Check sheet for the modelled part. Datum: model origin and axes. Units: mm. Face numbers are marked on the shaded views. A direction names the side the tool comes from. Give positions to 0.01 mm unless a question says otherwise; leave off trailing zeros. Write each loop counter-clockwise with the first axis right and the second up, starting at its lowest first coordinate (ties: lowest second). Pieces come first, ordered by that corner, then holes. Notation, with made-up numbers: (73, -0.5) -> (126, -0.5) arc R26 ccw to (126, 20.5) -> close; hole circle Ø7 at (-25, 89.25). An arc over 180 degrees is marked (long way). Answer as a JSON object with one key per item and string values.
from build123d import *

# Parameters (mm, degrees)
BOSS_EXTRUDE1_DEPTH = 19.05
SKETCH2_R           = 2
CUT_EXTRUDE1_DEPTH  = 10.16
SKETCH3_W           = 7.62
SKETCH3_H           = 3.81
CUT_EXTRUDE2_DEPTH  = 64.697811893


with BuildPart() as part:
    # Sketch1 → Boss-Extrude1 (new, symmetric)
    with BuildSketch(Plane.XY):
        with BuildLine():
            Line((-22.352, 0), (-22.352, 17.272))
            Line((-22.352, 17.272), (-19.812, 17.272))
            Line((-19.812, 17.272), (-19.812, 21.082))
            Line((-19.812, 21.082), (-28.702, 21.082))
            Line((-28.702, 21.082), (-28.702, 17.272))
            Line((-28.702, 17.272), (-26.162, 17.272))
            Line((-26.162, 17.272), (-26.162, 0))
            ThreePointArc((-26.162, 0), (0, -26.162), (26.162, 0))
            Line((26.162, 0), (26.162, 17.272))
            Line((26.162, 17.272), (28.702, 17.272))
            Line((28.702, 17.272), (28.702, 21.082))
            Line((28.702, 21.082), (19.812, 21.082))
            Line((19.812, 21.082), (19.812, 17.272))
            Line((19.812, 17.272), (22.352, 17.272))
            Line((22.352, 17.272), (22.352, 0))
            ThreePointArc((22.352, 0), (0, -22.352), (-22.352, 0))
        make_face()
    extrude(amount=BOSS_EXTRUDE1_DEPTH, both=True)

    # Sketch2 → Cut-Extrude1 (cut)
    with BuildSketch(Plane(origin=(0, 21.082, 0), x_dir=(1, 0, 0), z_dir=(0, 1, 0))):
        with Locations(Location((-24.257, 12.7, 0), (0, 0, 270))):
            Circle(SKETCH2_R)
        with Locations(Location((-24.257, -12.7, 0), (0, 0, 270))):
            Circle(SKETCH2_R)
        with Locations(Location((24.257, -12.7, 0), (0, 0, 270))):
            Circle(SKETCH2_R)
        with Locations(Location((24.257, 12.7, 0), (0, 0, 270))):
            Circle(SKETCH2_R)
    extrude(amount=-CUT_EXTRUDE1_DEPTH, mode=Mode.SUBTRACT)

    # Sketch3 → Cut-Extrude2 (cut, through all)
    with BuildSketch(Plane.ZY.offset(26.162)):
        with Locations((-12.7, 15.367)):
            Rectangle(SKETCH3_W, SKETCH3_H)
        with Locations((12.7, 15.367)):
            Rectangle(SKETCH3_W, SKETCH3_H)
    extrude(amount=-CUT_EXTRUDE2_DEPTH, mode=Mode.SUBTRACT)


solid = part.part
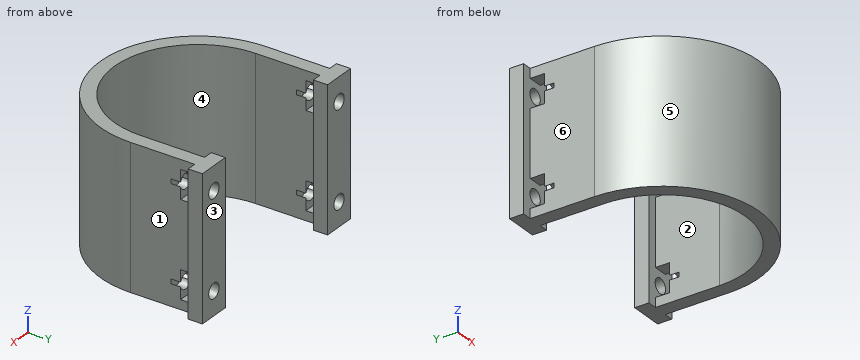
1. Sectioned sample at C-C, the plane x = -20.5. Enter the section's corners in (y, z).
Determined:
{"outline": "(-16.25, -19.05) -> (-8.91, -19.05) -> (-8.91, 19.05) -> (-16.25, 19.05) -> close; (17.27, -19.05) -> (21.08, -19.05) -> (21.08, 19.05) -> (17.27, 19.05) -> close"}
2. Access from +Z, -Z, +X, -X, +Y, -Y to the whole of each face (thin tool, end or side, straight path). Record for the marked faces 1, 2 and 3.
Determined:
{"face 1": "+Z, -Z, +X, -Y", "face 2": "+Z, -Z", "face 3": "+Z, -Z, +X, -X, +Y"}
3. Sectioned sample at A-A, the plane y = 6.5. Enter the section's corners in (x, z), plus the area to 3 significant figures.
Determined:
{"outline": "(-26.16, -19.05) -> (-22.35, -19.05) -> (-22.35, 19.05) -> (-26.16, 19.05) -> close; (22.35, -19.05) -> (26.16, -19.05) -> (26.16, 19.05) -> (22.35, 19.05) -> close", "area": "290 mm^2"}
4. Sectioned sample at D-D, the plane x = 0. Enter the section's corners in (y, z), plus the area to 3 significant figures.
Determined:
{"outline": "(-26.16, -19.05) -> (-22.35, -19.05) -> (-22.35, 19.05) -> (-26.16, 19.05) -> close", "area": "145 mm^2"}
5. Mould release check, pull along X, two halves, no side actions. Record for the marked faces 4, 5 and 6: released by +X, released by -X, zero draft, split by the parting line, or undercut.
Determined:
{"face 4": "undercut", "face 5": "split by the parting line", "face 6": "released by -X"}
6. Go/stop test with flat-tipped pins: P1, Ø4.5, axis at x = -26.5, z = 5, coming from the -Y side; P2, Ø6, axis at y = -18.5, z = -9.5, coming from the -X side; P3, Ø4.5, axis at x = 22, z = 7, coming from the -Y side. Record where each tip stops, or that it passes through.
Determined:
{"P1": "y = -9.82", "P2": "x = -21.08", "P3": "y = -17.16"}
7. Scan lines: L1, parallel to X at y = 20.3, z = 12.7; L2, parallel to X at y = 5, z = 12; L3, parallel to X at y = 19, z = 12. Record each from-to range of solid material in increasing order. Write a range as [from, to].
Determined:
{"L1": "[-28.7, -26.26], [-22.26, -19.81], [19.81, 22.26], [26.26, 28.7]", "L2": "[-26.16, -22.35], [22.35, 26.16]", "L3": "[-28.7, -26.13], [-22.38, -19.81], [19.81, 22.38], [26.13, 28.7]"}
8. Sectioned sample at B-B, the plane z = -15.5. Enter the section's corners in (x, y).
Determined:
{"outline": "(-28.7, 17.27) -> (-19.81, 17.27) -> (-19.81, 21.08) -> (-28.7, 21.08) -> close; (-26.16, 0) arc R26.16 ccw to (26.16, 0) -> (26.16, 13.46) -> (22.35, 13.46) -> (22.35, 0) arc R22.35 cw to (-22.35, 0) -> (-22.35, 13.46) -> (-26.16, 13.46) -> close; (19.81, 17.27) -> (28.7, 17.27) -> (28.7, 21.08) -> (19.81, 21.08) -> close"}
